Build history of the part. All positions in model axes, mm. A direction names the side the tool comes from. Round coordinates to 2 decimals unless told otherwise and drop trailing zeros. Loops run counter-clockwise (first coordinate to the right, second up) from the corner with the lowest first, then second, coordinate; pieces in that order, holes last. Notation, with made-up numbers: (-19.75, 53.5) - (32.25, 53.5) arc R16 ccw to (32.25, 69.5) - close; hole circle Ø8 at (86.5, 63). An arc over 180 degrees is marked (long way). Put each result on its own line as item: value. Start each with the question number.
from build123d import *

# Parameters (mm, degrees)
F1_DEPTH = 6.35
F2_DEPTH = 6.35
F2_TAPER = 30
F3_R     = 6.35
F4_DEPTH = 25.4
F5_W     = 51.275
F5_H     = 51.275
F5_W_2   = 41.275
F5_H_2   = 41.275
F6_DEPTH = 2.54


with BuildPart() as f1:
    # F0 (on Top) → F1 (new body)
    with BuildSketch(Plane.XY):
        with BuildLine():
            Line((64.1179559298, 56.275), (25.6375, 56.275))
            Line((25.6375, 56.275), (-12.8429559298, 56.275))
            ThreePointArc((-12.8429559298, 56.275), (-17.9816380777, 53.6554752757), (-18.8806651275, 47.95813253))
            Line((-18.8806651275, 47.95813253), (-1.4278661837, -5.61686747))
            ThreePointArc((-1.4278661837, -5.61686747), (0.8793677383, -8.7886821479), (4.609843014, -10))
            Line((4.609843014, -10), (18.1375, -10))
            Line((18.1375, -10), (10.4500775472, 39.1765561679))
            ThreePointArc((10.4500775472, 39.1765561679), (11.3197051539, 42.2423099321), (14.2143615238, 43.575))
            Line((14.2143615238, 43.575), (37.0606384762, 43.575))
            ThreePointArc((37.0606384762, 43.575), (39.9552948461, 42.2423099321), (40.8249224528, 39.1765561679))
            Line((40.8249224528, 39.1765561679), (33.1375, -10))
            Line((33.1375, -10), (46.665156986, -10))
            ThreePointArc((46.665156986, -10), (50.3956322617, -8.7886821479), (52.7028661837, -5.61686747))
            Line((52.7028661837, -5.61686747), (70.1556651275, 47.95813253))
            ThreePointArc((70.1556651275, 47.95813253), (69.2566380777, 53.6554752757), (64.1179559298, 56.275))
        make_face()
        with BuildLine():
            Line((10.4500775472, 39.1765561679), (18.1375, -10))
            Line((18.1375, -10), (25.6375, -10))
            Line((25.6375, -10), (33.1375, -10))
            Line((33.1375, -10), (40.8249224528, 39.1765561679))
            ThreePointArc((40.8249224528, 39.1765561679), (39.9552948461, 42.2423099321), (37.0606384762, 43.575))
            Line((37.0606384762, 43.575), (14.2143615238, 43.575))
            ThreePointArc((14.2143615238, 43.575), (11.3197051539, 42.2423099321), (10.4500775472, 39.1765561679))
        make_face()
    extrude(amount=-F1_DEPTH)

    # F0 (on Top) → F2 (join)
    with BuildSketch(Plane.XY):
        with BuildLine():
            Line((64.1179559298, 56.275), (25.6375, 56.275))
            Line((25.6375, 56.275), (-12.8429559298, 56.275))
            ThreePointArc((-12.8429559298, 56.275), (-17.9816380777, 53.6554752757), (-18.8806651275, 47.95813253))
            Line((-18.8806651275, 47.95813253), (-1.4278661837, -5.61686747))
            ThreePointArc((-1.4278661837, -5.61686747), (0.8793677383, -8.7886821479), (4.609843014, -10))
            Line((4.609843014, -10), (18.1375, -10))
            Line((18.1375, -10), (10.4500775472, 39.1765561679))
            ThreePointArc((10.4500775472, 39.1765561679), (11.3197051539, 42.2423099321), (14.2143615238, 43.575))
            Line((14.2143615238, 43.575), (37.0606384762, 43.575))
            ThreePointArc((37.0606384762, 43.575), (39.9552948461, 42.2423099321), (40.8249224528, 39.1765561679))
            Line((40.8249224528, 39.1765561679), (33.1375, -10))
            Line((33.1375, -10), (46.665156986, -10))
            ThreePointArc((46.665156986, -10), (50.3956322617, -8.7886821479), (52.7028661837, -5.61686747))
            Line((52.7028661837, -5.61686747), (70.1556651275, 47.95813253))
            ThreePointArc((70.1556651275, 47.95813253), (69.2566380777, 53.6554752757), (64.1179559298, 56.275))
        make_face()
    extrude(amount=F2_DEPTH, taper=F2_TAPER)

    # F3 (on face) → F4 (cut)
    with BuildSketch(Plane.XY):
        with Locations((25.6375, 34.05)):
            Circle(F3_R)
    extrude(amount=-F4_DEPTH, mode=Mode.SUBTRACT)

    # F5 (on face) → F6 (cut)
    with BuildSketch(Plane(origin=(0, 0, -6.35), x_dir=(1, 0, 0), z_dir=(0, 0, -1))):
        with Locations((25.6375, -25.6375)):
            Rectangle(F5_W, F5_H)
        with Locations((25.6375, -25.6375)):
            Rectangle(F5_W_2, F5_H_2, mode=Mode.SUBTRACT)
    extrude(amount=-F6_DEPTH, mode=Mode.SUBTRACT)


solid = f1.part
1) Pull direction X, two halves, no side cores. Call faces 1 (the face through (48, 25, -3.81)), 2 (the face through (49.3, -7.3, 3.2)), 3 (the face through (7, 30, 6.35)): pulls with the +X half, pulls with the -X half, needs draft (parallel to the pull), parting line crosses it, or undercut.
2) Which spindle directions (+Z, -Z, +X, -X, +Y, -Y) get a long thin tool onto all of the face, cutting with end or side? Do faces 4 (the face through (69.305, 53.587, -3.131)), 5 (the face through (0, 26, -5)), 6 (the face through (38.7, 14, 3.1)). Say none if no direction does.
3) Slice it at B-B, the plane y = 29.5. Write the cut outline in (x, z) (3 decimals), and give its area (3 significant figures).
4) Drop flat-ended pins along their axis: pin 1 Ø6 at (y, z) = (-2.5, -5) entering from +X; pin 2 Ø0.8 at (y, z) = (28.5, -4.5) entering from -X; pin 3 Ø20.5 at (x, y) = (25.64, 34.05) entering from -Z; pin 4 Ø2 at (y, z) = (22, -5) entering from +X. Give the stop position or say it passes through.
5) Slice it at C-C, the plane z = 3.25. Write the cut outline in (x, y) (3 decimals), and give its area (3 significant figures).
6) Drill centre lines: line 1 (Z direction, x = 50, y = 30.5); line 2 (X direction, y = 32, z = -3.75); line 3 (Y direction, x = 30.5, z = -1.5) (3 decimals). Where is each one in solid material? Low to high. Write a range as [from, to].
7) Slice it at D-D, the plane x = -5. Write the cut outline in (y, z) (3 decimals).
8) Slice it at A-A, the plane z = -5. State how many separate pieces and enclosed holes the cut face has, and give its area (3 significant figures).
Taken from the geometry:
1. face 1: undercut
1. face 2: pulls with the +X half
1. face 3: needs draft
2. face 4: +Z, -Z, +X
2. face 5: -Z
2. face 6: +Z
3. outline: (-12.868, -6.35) - (0, -6.35) - (0, -3.81) - (5, -3.81) - (5, -6.35) - (21.208, -6.35) - (21.208, 0) - (11.963, 0) - (8.252, 6.35) - (-9.012, 6.35) - (-12.868, 0) - close; (30.067, -6.35) - (46.275, -6.35) - (46.275, -3.81) - (51.275, -3.81) - (51.275, -6.35) - (64.143, -6.35) - (64.143, 0) - (60.287, 6.35) - (43.023, 6.35) - (39.312, 0) - (30.067, 0) - close
3. area: 675 mm2
4. pin 1: stops at x = 54.7
4. pin 2: stops at x = -12.67
4. pin 3: stops at z = -6.35
4. pin 4: stops at x = 62.03
5. outline: (-17.097, 48.539) - (0.356, -5.036) arc R4.474 ccw to (4.61, -8.124) - (15.945, -8.124) - (8.596, 38.887) arc R5.686 cw to (14.214, 45.451) - (37.061, 45.451) arc R5.686 cw to (42.679, 38.887) - (35.33, -8.124) - (46.665, -8.124) arc R4.474 ccw to (50.919, -5.036) - (68.372, 48.539) arc R4.474 ccw to (64.118, 54.399) - (-12.843, 54.399) arc R4.474 ccw to start
5. area: 2,820 mm2
6. line 1: z = [-3.81, 6.35]
6. line 2: x = [-13.68, 19.63], [31.65, 64.96]
6. line 3: y = [-10, 29.966], [38.134, 56.275]
7. outline: (5.349, -6.35) - (56.275, -6.35) - (56.275, 0) - (52.609, 6.35) - (17.185, 6.35) - (5.349, 0) - close
8. separate pieces: 2
8. enclosed holes: 2
8. area: 3,730 mm2
